from build123d import *

# Parameters (mm, degrees)
SKETCH_1_W      = 400
SKETCH_1_H      = 250
EXTRUDE_1_DEPTH = 80
SKETCH_3_R      = 26.348031195
EXTRUDE_2_DEPTH = 10
SKETCH_2_R      = 25.309072204
EXTRUDE_3_DEPTH = 10


with BuildPart() as part:
    # 草图1 → 凸台-拉伸1 (new body)
    with BuildSketch(Plane(origin=(0, 0, 0), x_dir=(1, 0, 0), z_dir=(0, 1, 0))):
        with Locations((10.638297872, -13.031914894)):
            Rectangle(SKETCH_1_W, SKETCH_1_H)
    extrude(amount=EXTRUDE_1_DEPTH)

    # 草图3 → 凸台-拉伸2 (add)
    with BuildSketch(Plane(origin=(0, 0, -111.968085106), x_dir=(-1, 0, 0), z_dir=(0, 0, -1))):
        with Locations(Location((-10.638297872, 40, 0), (0, 0, 180))):
            Circle(SKETCH_3_R)
    extrude(amount=EXTRUDE_2_DEPTH)

    # 草图2 → 凸台-拉伸3 (add)
    with BuildSketch(Plane.XY.offset(138.031914894)):
        with Locations(Location((-150.390563376, 40, 0), (0, 0, 180))):
            Circle(SKETCH_2_R)
        with Locations(Location((-50.390563376, 40, 0), (0, 0, 180))):
            Circle(SKETCH_2_R)
        with Locations(Location((49.609436624, 40, 0), (0, 0, 180))):
            Circle(SKETCH_2_R)
        with Locations(Location((149.609436624, 40, 0), (0, 0, 180))):
            Circle(SKETCH_2_R)
    extrude(amount=EXTRUDE_3_DEPTH)


solid = part.part
Model file for the job. Use its own axes, mm. A direction names the side the tool comes from. Coordinates: 2 decimals unless noted, no trailing zeros. Order: outer loops, then holes, each group sorted by start corner. A loop starts at its lowest first (then second) coordinate and runs counter-clockwise, first axis right, second up. Notation, with made-up numbers: (70.25, -5) -> (77.25, -5) arc R16 cw to (77.25, 0) -> close; hole circle Ø6 at (28, -11). An arc over 180 degrees is marked (long way). Return JSON: item names as keys, results as strings. Group by question number.
Item 1: Saw through at A-A on y = 40. Write the cut outline in (x, z).
Item 2: Tool access for faces 1 (the flat face through (50, 40, 148.032)), 2 (the cylindrical face through (-125.106, 38.887, 142.962)), 3 (the cylindrical face through (7.208, 13.876, -116.898)): list every direction of +Z, -Z, +X, -X, +Y, -Y with a clear straight run to the whole face (end or side of a thin tool).
Item 3: Saw through at D-D on y = 61. Write the cut outline in (x, z).
Item 4: Saw through at B-B on x = -152. Write the cut outline in (y, z), then the cut area to 3 significant figures.
Item 5: Wall check: line 1 along Z through (x, y) = (137, 21); line 2 along Z through (x, y) = (-94, 36). Give the ranges that are in metal, low to high. Write a range as [from, to].
Item 6: Saw through at C-C on x = 14.5. Write the cut outline in (y, z), then the cut area to 3 significant figures.
Item 7: Flat gauge pins, fed straight in: P1, Ø3, axis at x = -92.5, y = 38, coming from the -Z side; P2, Ø1, axis at x = -76.5, z = 7.5, coming from the -Y side; P3, Ø1.5, axis at x = 141.5, y = 70, coming from the +Z side. Where does each tip first touch, or does it go through?
Values found:
{
 "1": {"outline": "(-189.36, -111.97) -> (-15.71, -111.97) -> (-15.71, -121.97) -> (36.99, -121.97) -> (36.99, -111.97) -> (210.64, -111.97) -> (210.64, 138.03) -> (174.92, 138.03) -> (174.92, 148.03) -> (124.3, 148.03) -> (124.3, 138.03) -> (74.92, 138.03) -> (74.92, 148.03) -> (24.3, 148.03) -> (24.3, 138.03) -> (-25.08, 138.03) -> (-25.08, 148.03) -> (-75.7, 148.03) -> (-75.7, 138.03) -> (-125.08, 138.03) -> (-125.08, 148.03) -> (-175.7, 148.03) -> (-175.7, 138.03) -> (-189.36, 138.03) -> close"},
 "2": {"face 1": "+Z, +X, -X, +Y, -Y", "face 2": "+Z", "face 3": "-Z"},
 "3": {"outline": "(-189.36, -111.97) -> (-5.27, -111.97) -> (-5.27, -121.97) -> (26.55, -121.97) -> (26.55, -111.97) -> (210.64, -111.97) -> (210.64, 138.03) -> (163.74, 138.03) -> (163.74, 148.03) -> (135.48, 148.03) -> (135.48, 138.03) -> (63.74, 138.03) -> (63.74, 148.03) -> (35.48, 148.03) -> (35.48, 138.03) -> (-36.26, 138.03) -> (-36.26, 148.03) -> (-64.52, 148.03) -> (-64.52, 138.03) -> (-136.26, 138.03) -> (-136.26, 148.03) -> (-164.52, 148.03) -> (-164.52, 138.03) -> (-189.36, 138.03) -> close"},
 "4": {"outline": "(0, -111.97) -> (80, -111.97) -> (80, 138.03) -> (65.26, 138.03) -> (65.26, 148.03) -> (14.74, 148.03) -> (14.74, 138.03) -> (0, 138.03) -> close", "area": "20,500 mm2"},
 "5": {"line 1": "z = [-111.97, 148.03]", "line 2": "z = [-111.97, 138.03]"},
 "6": {"outline": "(0, -111.97) -> (13.94, -111.97) -> (13.94, -121.97) -> (66.06, -121.97) -> (66.06, -111.97) -> (80, -111.97) -> (80, 138.03) -> (0, 138.03) -> close", "area": "20,500 mm2"},
 "7": {"P1": "stops at z = -111.97", "P2": "stops at y = 0", "P3": "stops at z = 138.03"}
}
